Design review of the part built by this model. Coordinates are the model's own, in mm. Face numbers are marked on the shaded views. A direction names the side the tool comes from. Round coordinates to 2 decimals unless told otherwise and drop trailing zeros. Loops run counter-clockwise (first coordinate to the right, second up) from the corner with the lowest first, then second, coordinate; pieces in that order, holes last. Notation, with made-up numbers: (49, 80.5) -> (68, 80.5) arc R17 cw to (68, 92.5) -> close; hole circle Ø7 at (80, 39.5). An arc over 180 degrees is marked (long way). Answer as CSV lines item,"result". Start each with the question number.
(1) Take a section at C-C, the plane y = 26. Write out the cut boundary in (x, z).
(2) For P1, Ø12, axis at x = 35.5, y = 62, coming from the +Z side; P2, Ø0.6, axis at x = 0.5, y = 56.5, coming from the -Z side; P3, Ø0.6, axis at x = 1, z = 13, coming from the -Y side; P4, Ø1.5, axis at y = 65.5, z = 12, coming from the -X side, all flat-tipped, find the tip position at first contact; note any pin that passes through.
(3) Machinability: for the marked faces 1, 2 and 3, which of the approach directions +Z, -Z, +X, -X, +Y, -Y give a long, thin tool a straight path to every point of the face, cutting with its end or side? Answer none if there is none.
(4) Take a section at B-B, the plane x = 31. Write out the cut boundary in (y, z).
(5) Take a section at A-A, the plane y = 64.5. Write out the cut boundary in (x, z), and give its area (3 significant figures).
(6) Draft analysis for pull direction Z (two halves, no side actions). For the marked faces 4, 5 and 6, state which applies: +Z half, -Z half, draft (parallel to the pull), parting line (faces both ways), or undercut.
(7) To check wall thickness, follow line 1 (X direction, y = 14.5, z = 12.25); line 2 (Z direction, x = 0.8, y = 39); line 3 (X direction, y = 56, z = 16.75). State the ranges of each line that lie inside material, in increasing order. Write a range as from..to.
(8) Take a section at D-D, the plane x = 22.5. Write out the cut boundary in (y, z).
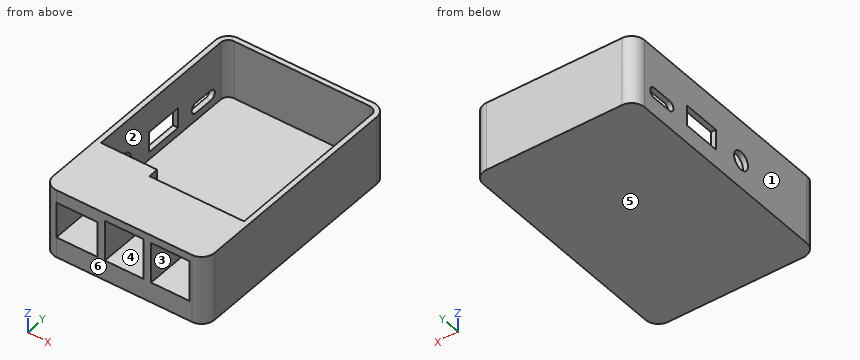
from build123d import *

# Parameters (mm, degrees)
BOSS_EXTRU_1_DEPTH      = 27
ESQUISSE2_R             = 3.6
ESQUISSE2_W             = 8
ESQUISSE2_H             = 15
ENL_V_MAT_EXTRU_1_DEPTH = 9
ESQUISSE3_W             = 16
ESQUISSE3_H             = 14
ESQUISSE3_W_2           = 15
ESQUISSE3_H_2           = 16
ENL_V_MAT_EXTRU_2_DEPTH = 19
ENL_V_MAT_EXTRU_3_DEPTH = 23


with BuildPart() as part:
    # Esquisse1 → Boss.-Extru.1 (new body)
    with BuildSketch(Plane.XY):
        with BuildLine():
            Line((5, 0), (58, 0))
            ThreePointArc((58, 0), (61.535533906, 1.464466094), (63, 5))
            Line((63, 5), (63, 89))
            ThreePointArc((63, 89), (61.535533906, 92.535533906), (58, 94))
            Line((58, 94), (5, 94))
            ThreePointArc((5, 94), (1.464466094, 92.535533906), (0, 89))
            Line((0, 89), (0, 5))
            ThreePointArc((0, 5), (1.464466094, 1.464466094), (5, 0))
        make_face()
    extrude(amount=BOSS_EXTRU_1_DEPTH)

    # Esquisse2 → Enlèv. mat.-Extru.1 (cut)
    with BuildSketch(Plane.ZY):
        with Locations(Location((11, 39, 0), (0, 0, 270))):
            Circle(ESQUISSE2_R)
        with BuildLine():
            Line((11, 84), (11, 76))
            ThreePointArc((11, 76), (9, 74), (7, 76))
            Line((7, 76), (7, 84))
            ThreePointArc((7, 84), (9, 86), (11, 84))
        make_face()
        with Locations((11, 59.5)):
            Rectangle(ESQUISSE2_W, ESQUISSE2_H)
    extrude(amount=-ENL_V_MAT_EXTRU_1_DEPTH, mode=Mode.SUBTRACT)

    # Esquisse3 → Enlèv. mat.-Extru.2 (cut)
    with BuildSketch(Plane.XZ):
        with Locations((13, 15)):
            Rectangle(ESQUISSE3_W, ESQUISSE3_H)
        with Locations((31.5, 16)):
            Rectangle(ESQUISSE3_W_2, ESQUISSE3_H_2)
        with Locations((49.5, 16)):
            Rectangle(ESQUISSE3_W_2, ESQUISSE3_H_2)
    extrude(amount=-ENL_V_MAT_EXTRU_2_DEPTH, mode=Mode.SUBTRACT)

    # Esquisse4 → Enlèv. mat.-Extru.3 (cut)
    with BuildSketch(Plane.XY.offset(27)):
        with BuildLine():
            Line((2, 27), (24, 27))
            Line((24, 27), (24, 23))
            Line((24, 23), (61, 23))
            Line((61, 23), (61, 27))
            Line((61, 27), (61, 89))
            ThreePointArc((61, 89), (60.121320344, 91.121320344), (58, 92))
            Line((58, 92), (5, 92))
            ThreePointArc((5, 92), (2.878679656, 91.121320344), (2, 89))
            Line((2, 89), (2, 27))
        make_face()
    extrude(amount=-ENL_V_MAT_EXTRU_3_DEPTH, mode=Mode.SUBTRACT)


solid = part.part
The answers:
1,outline,"(0, 0) -> (63, 0) -> (63, 27) -> (61, 27) -> (61, 4) -> (24, 4) -> (24, 27) -> (0, 27) -> close"
2,P1,"z = 4"
2,P2,"z = 0"
2,P3,"y = 1.64"
2,P4,"x = 61"
3,face 1,"+Z, -Z, -X, +Y, -Y"
3,face 2,"+Z"
3,face 3,"-Y"
4,outline,"(0, 0) -> (94, 0) -> (94, 27) -> (92, 27) -> (92, 4) -> (23, 4) -> (23, 27) -> (0, 27) -> (0, 24) -> (19, 24) -> (19, 8) -> (0, 8) -> close"
5,outline,"(0, 0) -> (63, 0) -> (63, 27) -> (61, 27) -> (61, 4) -> (2, 4) -> (2, 7) -> (0, 7) -> close; (0, 15) -> (2, 15) -> (2, 27) -> (0, 27) -> close"
5,area,"328 mm²"
6,face 4,"undercut"
6,face 5,"-Z half"
6,face 6,"draft"
7,line 1,"0..5, 21..24, 39..42, 57..63"
7,line 2,"0..7.4, 14.6..27"
7,line 3,"0..2, 61..63"
8,outline,"(0, 0) -> (94, 0) -> (94, 27) -> (92, 27) -> (92, 4) -> (27, 4) -> (27, 27) -> (0, 27) -> close"
